CAD build for the part. Positions are in the model's coordinates, mm. Face numbers are marked on the shaded views. A direction names the side the tool comes from. Give positions to 0.01 mm unless a question says otherwise; leave off trailing zeros. Order: outer loops, then holes, each group sorted by start corner. A loop starts at its lowest first (then second) coordinate and runs counter-clockwise, first axis right, second up.
Autodesk Inventor part; units mm, degrees
ref_plane "YZ Plane" through (0, 0, 0) normal (1, 0, 0) x (0, 1, 0)
ref_plane "XZ Plane" through (0, 0, 0) normal (0, 1, 0) x (-1, 0, 0)
ref_plane "XY Plane" through (0, 0, 0) normal (0, 0, 1) x (1, 0, 0)
sketch "Sketch1" plane through (0, 0, 0) normal (0, 0, 1) x (1, 0, 0)
  line L0 (0, 0) -> (2.5, 0)
  line L1 (2.5, 0) -> (2.5, 45)
  line L2 (2.5, 45) -> (-2.5, 45)
  line L3 (-2.5, 45) -> (-2.5, 0)
  circle A0 centre (0, 0) radius 8.5
  line L4 (0, 45) -> (8.5, 45) construction
  circle A1 centre (0, 45) radius 8.5
  line L5 (-8.5, 0) -> (-8.5, 45)
  line L6 (8.5, 45) -> (8.5, 0)
  line L7 (0, 45) -> (8.5, 45)
  line L8 (0, 45) -> (-8.5, 36.5)
  line L9 (0, 45) -> (12.0208, 45) construction
  line L10 (0, 0) -> (8.5, 0)
  line L11 (0, 0) -> (-8.5, 8.5)
  line L12 (0, 0) -> (12.0208, 0) construction
  dimension "d9" = 17
  dimension "d1" = 2.5
  dimension "d2" = 45
  dimension "d3" = 5
  dimension "d5" = 17
  dimension "d10" = 2.5
  dimension "d11" = 0
  dimension "d12" = 135
  dimension "d13" = 135
extrude "Extrusion1" add sketch "Sketch1" along normal blind 20 contours L11 L3 A0 L1 L0 | L1 A0 L10 | L11 A0 L3 | A0 L3 A1 L1 | L1 A1 L6 A0 | A0 L11 L5 L8 A1 L3 | A1 L3 L8 L2 L1 | L1 L7 A1 | A1 L8 L3
sketch "Sketch2" plane through (0, 0, 0) normal (0, 0, -1) x (-1, 0, 0)
  line L0 (0, 0) -> (-8.5, 0)
  line L1 (0, 0) -> (0, 8)
  circle A0 centre (0, 8) radius 2.5
  line L2 (8.5, 8.5) -> (0, 0)
  line L3 (0, 0) -> (-1.5, 0)
  line L4 (-1.5, 0) -> (-1.5, 8)
  line L5 (-1.5, 8) -> (1.5, 8)
  line L6 (1.5, 8) -> (1.5, 0)
  line L7 (1.5, 0) -> (0, 0)
  line L8 (0, 45) -> (8.5, 36.5)
  line L9 (0, 45) -> (0, 37)
  line L10 (0, 37) -> (-1.5, 37)
  line L11 (-1.5, 37) -> (-1.5, 45)
  line L12 (-8.5, 45) -> (0, 45)
  line L13 (0, 37) -> (1.5, 37)
  line L14 (1.5, 37) -> (1.5, 45)
  line L15 (1.5, 45) -> (0, 45)
  circle A1 centre (0, 37) radius 2.5
  point P0 (-1.5, 39)
  point P1 (1.5, 39)
  point P2 (-1.5, 6)
  point P3 (1.5, 6)
  dimension "d16" = 8
  dimension "d17" = 5
  dimension "d18" = 1.5
  dimension "d19" = 3
  dimension "d20" = 8
  dimension "d21" = 1.5
  dimension "d22" = 1.5
  dimension "d23" = 5
extrude "Extrusion2" cut sketch "Sketch2" against normal through all
fillet "Fillet1" radius 8 4 edges at (8.5, 22.5, 0) (8.5, 22.5, 20) (-8.5, 22.5, 0) (-8.5, 22.5, 20)
sketch "Sketch4" plane through (1.5, 0, 0.0627) normal (0, -1, 0) x (1, 0, 0)
  line L0 (-10, 7.9373) -> (-10, 11.9373)
  line L1 (-10, 9.9373) -> (-8, 9.9373)
  circle A0 centre (-8, 9.9373) radius 1
  point P0 (-1.5, -0.0627)
  dimension "d31" = 2
  dimension "d32" = 2
extrude "Extrusion4" cut sketch "Sketch4" against normal through all
properties part number "index_f1"
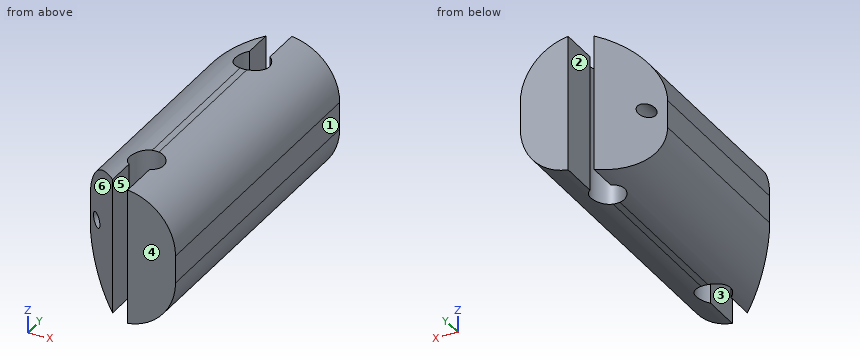
1. Saw through at C-C on y = 37. Give the cut face in (x, z).
2. Wall check: line 1 (X direction, y = 16.5, z = 10); line 2 (Y direction, x = 0, z = 15); line 3 (Y direction, x = -2.25, z = 9). Give the ranges that are in metal, low to high.
3. Mould opens along X. For the marked faces 4, 5 and 6 say: released by +X, released by -X, zero draft, split by the parting line, or undercut.
4. Saw through at A-A on y = 29. Give the cut face in (x, z).
5. Pin check, flat tips, straight feed: P1, Ø5, axis at y = 27, z = 4, coming from the -X side; P2, Ø4.5, axis at x = 0, y = 37, coming from the -Z side; P3, Ø5, axis at y = 3, z = 7, coming from the +X side; P4, Ø6.5, axis at y = 3, z = 10, coming from the -X side. Stop position of each tip, or through.
6. Saw through at B-B on z = 10. Give the cut face in (x, y).
7. Saw through at D-D on x = -6.5. Give the cut face in (y, z).
8. 3-axis set-ups, long thin cutter, end or side, ignore diameter. For the marked faces 1, 2 and 3: which of +Z, -Z, +X, -X, +Y, -Y reach the whole face in a straight line?
Reported:
1. outline: (-8, 5.22) arc R8 ccw to (-2.5, 0.25) - (-2.5, 19.75) arc R8 ccw to (-8, 14.78) - close; (2.5, 0.25) arc R8 ccw to (8.5, 8) - (8.5, 12) arc R8 ccw to (2.5, 19.75) - close; hole circle Ø2 at (-6.5, 10)
2. line 1: x = -8.5 to -7.5, -5.5 to 8.5
2. line 2: y = 10.5 to 34.5
2. line 3: y = 2.25 to 6.91, 9.09 to 35.91, 38.09 to 42.75
3. face 4: zero draft
3. face 5: undercut
3. face 6: released by -X
4. outline: (-8.5, 8) arc R8 ccw to (-0.5, 0) - (0.5, 0) arc R8 ccw to (8.5, 8) - (8.5, 12) arc R8 ccw to (0.5, 20) - (-0.5, 20) arc R8 ccw to (-8.5, 12) - close; hole circle Ø2 at (-6.5, 10)
5. P1: stops at x = -8.36
5. P2: passes through
5. P3: stops at x = 8.5
5. P4: stops at x = -6.12
6. outline: (-8.5, 8.5) - (-7.5, 7.5) - (-7.5, 37.5) - (-8.5, 36.5) - close; (-5.5, 5.5) - (-1.5, 1.5) - (-1.5, 6) arc R2.5 cw (long way) to (1.5, 6) - (1.5, 0) - (8.5, 0) - (8.5, 45) - (1.5, 45) - (1.5, 39) arc R2.5 cw (long way) to (-1.5, 39) - (-1.5, 43.5) - (-5.5, 39.5) - close
7. outline: (6.5, 2.71) - (38.5, 2.71) - (38.5, 9) - (6.5, 9) - close; (6.5, 11) - (38.5, 11) - (38.5, 17.29) - (6.5, 17.29) - close
8. face 1: +Z, -Z, +X, +Y, -Y
8. face 2: +Z, -Z, +Y
8. face 3: +Z, -Z, -Y
